Geometry check sheet. Reference: the model listing, model coordinates, mm. A direction names the side the tool comes from. Coordinates: 2 decimals unless noted, no trailing zeros. Write each loop counter-clockwise with the first axis right and the second up, starting at its lowest first coordinate (ties: lowest second). Pieces come first, ordered by that corner, then holes. Notation, with made-up numbers: (36.25, 4.5) -> (49.25, 4.5) arc R8 cw to (49.25, 8.5) -> close; hole circle Ø10 at (76, -17). An arc over 180 degrees is marked (long way). Answer in a Markdown table with one row per item. Add a question column.
Q1. Section check A-A, the plane y = -9. Record the boundary of the cut face in (x, z), and give its area (3 significant figures).
Q2. Release check for a two-part mould opening along X. For faces 1 (the face through (35, 30, -1)), 2 (the face through (-23, 37, 2)), 3 (the face through (-52, -1, 2)) record: pulls with the +X half, pulls with the -X half, needs draft (parallel to the pull), parting line crosses it, or undercut.
Q3. Section check B-B, the plane z = 1.65. Count the separate pieces of the cut face and the enclosed holes in it, and give its area (3 significant figures).
Q4. Tool access check on faces 4 (the face through (35, -30, -1)), 5 (the face through (23, -41, 2)). Record the directions out of +Z, -Z, +X, -X, +Y, -Y that give a thin tool (end or side, any length) a straight path to the whole face; none if there is none.
Q5. Gauge pin test, flat ends, axial feed: P1, Ø2.5, axis at x = 12, y = 9, coming from the +Z side; P2, Ø1.2, axis at x = -22.5, y = 38.5, coming from the +Z side; P3, Ø3, axis at x = 0.5, y = -8.5, coming from the -Z side. Record the tip position at first contact, or that the pin passes through.
Q6. Section check C-C, the plane x = -11.5. Record the boundary of the cut face in (y, z), and give its area (3 significant figures).
Q7. Section check D-D, the plane y = 39. Record the boundary of the cut face in (x, z), and give its area (3 significant figures).
Q8. Thickness scan on line 1 (Y direction, x = 12, z = 3.5); line 2 (Y direction, x = -23, z = 1.6); line 3 (X direction, y = 20.5, z = 2). Record the ranges inside material, lowest first.
```python
from build123d import *

# Parameters (mm, degrees)
CROQUIS1_W              = 104
CROQUIS1_H              = 90
SALIENTE_EXTRUIR1_DEPTH = 5
CROQUIS3_W              = 34
CROQUIS3_H              = 30
SALIENTE_EXTRUIR2_DEPTH = 1
SKETCH1_R               = 2
CUT_EXTRUDE1_DEPTH      = 5


with BuildPart() as part:
    # Croquis1 → Saliente-Extruir1 (new body)
    with BuildSketch(Plane.XY):
        Rectangle(CROQUIS1_W, CROQUIS1_H)
    extrude(amount=SALIENTE_EXTRUIR1_DEPTH)

    # Croquis3 → Saliente-Extruir2 (add)
    with BuildSketch(Plane(origin=(0, 0, 0), x_dir=(-1, 0, 0), z_dir=(0, 0, -1))):
        with Locations((-35, 30)):
            Rectangle(CROQUIS3_W, CROQUIS3_H)
        with Locations((-35, -30)):
            Rectangle(CROQUIS3_W, CROQUIS3_H)
        with Locations((35, 30)):
            Rectangle(CROQUIS3_W, CROQUIS3_H)
        with Locations((35, -30)):
            Rectangle(CROQUIS3_W, CROQUIS3_H)
    extrude(amount=SALIENTE_EXTRUIR2_DEPTH)

    # Sketch1 → Cut-Extrude1 (cut)
    with BuildSketch(Plane(origin=(0, 0, 0), x_dir=(-1, 0, 0), z_dir=(0, 0, -1))):
        with Locations((-47, 39)):
            Circle(SKETCH1_R)
        with Locations((-23, 39)):
            Circle(SKETCH1_R)
        with Locations((-47, 21)):
            Circle(SKETCH1_R)
        with Locations((-23, 21)):
            Circle(SKETCH1_R)
        with Locations((23, 39)):
            Circle(SKETCH1_R)
        with Locations((23, 21)):
            Circle(SKETCH1_R)
        with Locations((47, 21)):
            Circle(SKETCH1_R)
        with Locations((47, 39)):
            Circle(SKETCH1_R)
        with Locations((23, -21)):
            Circle(SKETCH1_R)
        with Locations((23, -39)):
            Circle(SKETCH1_R)
        with Locations((47, -39)):
            Circle(SKETCH1_R)
        with Locations((47, -21)):
            Circle(SKETCH1_R)
        with Locations((-23, -21)):
            Circle(SKETCH1_R)
        with Locations((-23, -39)):
            Circle(SKETCH1_R)
        with Locations((-47, -39)):
            Circle(SKETCH1_R)
        with Locations((-47, -21)):
            Circle(SKETCH1_R)
        with Locations((-12, 9)):
            Circle(SKETCH1_R)
        with Locations((-12, -9)):
            Circle(SKETCH1_R)
        with Locations((12, -9)):
            Circle(SKETCH1_R)
        with Locations((12, 9)):
            Circle(SKETCH1_R)
    extrude(amount=-CUT_EXTRUDE1_DEPTH, mode=Mode.SUBTRACT)


solid = part.part
```
Calculated:
| question | item | result |
|---|---|---|
| 1 | outline | (-52, 0) -> (-14, 0) -> (-14, 5) -> (-52, 5) -> close; (-10, 0) -> (10, 0) -> (10, 5) -> (-10, 5) -> close; (14, 0) -> (52, 0) -> (52, 5) -> (14, 5) -> close |
| 1 | area | 480 mm² |
| 2 | face 1 | needs draft |
| 2 | face 2 | undercut |
| 2 | face 3 | pulls with the -X half |
| 3 | separate pieces | 1 |
| 3 | enclosed holes | 20 |
| 3 | area | 9,110 mm² |
| 4 | face 4 | -Z, +X, -X, +Y, -Y |
| 4 | face 5 | +Z |
| 5 | P1 | passes through |
| 5 | P2 | stops at z = 0 |
| 5 | P3 | stops at z = 0 |
| 6 | outline | (-45, 0) -> (-10.94, 0) -> (-10.94, 5) -> (-45, 5) -> close; (-7.06, 0) -> (7.06, 0) -> (7.06, 5) -> (-7.06, 5) -> close; (10.94, 0) -> (45, 0) -> (45, 5) -> (10.94, 5) -> close |
| 6 | area | 411 mm² |
| 7 | outline | (-52, -1) -> (-18, -1) -> (-18, 0) -> (18, 0) -> (18, -1) -> (52, -1) -> (52, 5) -> (49, 5) -> (49, 0) -> (45, 0) -> (45, 5) -> (25, 5) -> (25, 0) -> (21, 0) -> (21, 5) -> (-21, 5) -> (-21, 0) -> (-25, 0) -> (-25, 5) -> (-45, 5) -> (-45, 0) -> (-49, 0) -> (-49, 5) -> (-52, 5) -> close |
| 7 | area | 508 mm² |
| 8 | line 1 | y = -45 to -11, -7 to 7, 11 to 45 |
| 8 | line 2 | y = -45 to -41, -37 to -23, -19 to 19, 23 to 37, 41 to 45 |
| 8 | line 3 | x = -52 to -48.94, -45.06 to -24.94, -21.06 to 21.06, 24.94 to 45.06, 48.94 to 52 |
